from build123d import *

# Parameters (mm, degrees)
F1_W     = 161
F1_H     = 96
F1_H_2   = 2
F2_DEPTH = 30
F3_T     = -4
F4_W     = 161
F4_H     = 2
F4_W_2   = 2
F5_DEPTH = 100


with BuildPart() as f2:
    # F1 (on Front) → F2 (new body)
    with BuildSketch(Plane.XZ):
        Polygon((82.5, 50), (82.5, -50), (-82.5, -50), (-82.5, 50), (-84.5, 50), (-84.5, -52), (84.5, -52), (84.5, 50), align=None)
        Polygon((-82.5, -50), (82.5, -50), (82.5, 50), (80.5, 50), (80.5, 48), (80.5, -48), (-80.5, -48), (-80.5, 48), (-80.5, 50), (-82.5, 50), align=None)
        Rectangle(F1_W, F1_H)
        with Locations((0, 49)):
            Rectangle(F1_W, F1_H_2)
    extrude(amount=-F2_DEPTH)

    # F3
    f3_openings = [f2.faces().sort_by_distance(p)[0] for p in [
        (0, 15, 50),
        (0, 0, -1),
    ]]
    offset(amount=F3_T, openings=f3_openings)

    # F4 (on face) → F5 (cut)
    with BuildSketch(Plane.XY.offset(50)):
        with Locations((0, 3)):
            Rectangle(F4_W, F4_H)
        with Locations((-81.5, 3)):
            Rectangle(F4_W_2, F4_H)
        with Locations((81.5, 3)):
            Rectangle(F4_W_2, F4_H)
    extrude(amount=-F5_DEPTH, mode=Mode.SUBTRACT)


solid = f2.part
Geometry check sheet. Reference: the model listing, model coordinates, mm. A direction names the side the tool comes from. Give positions to 0.01 mm unless a question says otherwise; leave off trailing zeros. Loops run counter-clockwise (first coordinate to the right, second up) from the corner with the lowest first, then second, coordinate; pieces in that order, holes last.
(1) Release check for a two-part mould opening along X. For faces 3 (the flat face through (-84.5, 15, 0)), 4 (the flat face through (-1, 30, 0)), 5 (the flat face through (84.5, 15, -2)), 6 (the flat face through (80.5, 15, 0)) record: released by +X, released by -X, zero draft, split by the parting line, or undercut.
From the geometry:
face 3: released by -X
face 4: zero draft
face 5: released by +X
face 6: undercut
(2) Depth check by flat-ended pin: pin 1 Ø4 at (x, z) = (-28.5, 3) entering from -Y; pin 2 Ø2 at (x, y) = (-61, 8) entering from +Z. Enter the tip coordinate at first touch or a pass-through.
From the geometry:
pin 1: stops at y = 26
pin 2: stops at z = -48
(3) Set-up check for faces 1 (the flat face through (0, 27, 50)), 2 (the flat face through (-1, 26, 2)): record each of +Z, -Z, +X, -X, +Y, -Y from which the full face is reachable in a straight line by a thin tool's end or side.
From the geometry:
face 1: +Z, +X, -X, +Y, -Y
face 2: +Z, -Y
(4) Section check C-C on z = 38.5. Record the cut outline in (x, y), then the cut area to 3 significant figures.
From the geometry:
outline: (-84.5, 0) - (-80.5, 0) - (-80.5, 2) - (-82.5, 2) - (-82.5, 4) - (-80.5, 4) - (-80.5, 26) - (80.5, 26) - (80.5, 4) - (82.5, 4) - (82.5, 2) - (80.5, 2) - (80.5, 0) - (84.5, 0) - (84.5, 30) - (-84.5, 30) - close
area: 876 mm2
(5) Section check B-B on x = 62. Record the cut outline in (y, z).
From the geometry:
outline: (0, -52) - (30, -52) - (30, 50) - (26, 50) - (26, -48) - (4, -48) - (4, -50) - (2, -50) - (2, -48) - (0, -48) - close
(6) Section check A-A on y = 21.5. Record the cut outline in (x, z).
From the geometry:
outline: (-84.5, -52) - (84.5, -52) - (84.5, 50) - (80.5, 50) - (80.5, -48) - (-80.5, -48) - (-80.5, 50) - (-84.5, 50) - close
(7) Thickness scan on L1, parallel to X at y = 25.5, z = 0; L2, parallel to X at y = 3.75, z = 23; L3, parallel to Y at x = -53, z = 19.5. Record the ranges inside material, lowest first.
From the geometry:
L1: x = -84.5 to -80.5, 80.5 to 84.5
L2: x = -84.5 to -82.5, 82.5 to 84.5
L3: y = 26 to 30
